Read the model definition and answer for the solid it produces. Units are mm, in the model's axes. A direction names the side the tool comes from. Give positions to 0.01 mm unless a question says otherwise; leave off trailing zeros. Write each loop counter-clockwise with the first axis right and the second up, starting at its lowest first coordinate (ties: lowest second). Pieces come first, ordered by that corner, then holes. Notation, with made-up numbers: M 5,-37 L 9,-37 A22 ccw 9,-25 Z; hole C -1.75,25.5 d2. An arc over 180 degrees is marked long. Write each question's results on one line, items separated by ' | '. Start each with the question number.
```python
from build123d import *

# Parameters (mm, degrees)
SKETCH1_R           = 2.413
SKETCH1_R_2         = 2.38125
SKETCH1_W           = 12.7
SKETCH1_H           = 3.81
BOSS_EXTRUDE1_DEPTH = 3.175
SKETCH3_W           = 292.1
SKETCH3_H           = 12.573
BOSS_EXTRUDE2_DEPTH = 8.89
BOSS_EXTRUDE3_DEPTH = 4.1275
FILLET1_R           = 2.54
FILLET2_R           = 1.27


with BuildPart() as part:
    # Sketch1 → Boss-Extrude1 (new, symmetric)
    with BuildSketch(Plane.XY):
        Polygon((-292.1, -6.2865), (-12.7, -6.2865), (-12.7, -19.05), (0, -19.05), (0, 19.05), (-12.7, 19.05), (-12.7, 6.2865), (-292.1, 6.2865), (-292.1, 8.8265), (-304.8, 19.05), (-314.96, 19.05), (-314.96, -19.05), (-304.8, -19.05), (-292.1, -8.8265), align=None)
        with Locations((-309.88, -12.7)):
            Circle(SKETCH1_R, mode=Mode.SUBTRACT)
        with Locations(Location((-309.88, 12.7, 0), (0, 0, 180))):
            Circle(SKETCH1_R, mode=Mode.SUBTRACT)
        with Locations((-6.35, 12.7)):
            Circle(SKETCH1_R_2, mode=Mode.SUBTRACT)
        with Locations(Location((-6.35, -12.7, 0), (0, 0, 180))):
            Circle(SKETCH1_R_2, mode=Mode.SUBTRACT)
        with Locations((-300.99, 3.81)):
            Rectangle(SKETCH1_W, SKETCH1_H, mode=Mode.SUBTRACT)
        with Locations((-300.99, -3.81)):
            Rectangle(SKETCH1_W, SKETCH1_H, mode=Mode.SUBTRACT)
    extrude(amount=BOSS_EXTRUDE1_DEPTH, both=True)

    # Sketch3 → Boss-Extrude2 (add)
    with BuildSketch(Plane(origin=(0, 0, -3.175), x_dir=(-1, 0, 0), z_dir=(0, 0, -1))):
        with Locations((146.05, 0)):
            Rectangle(SKETCH3_W, SKETCH3_H)
    extrude(amount=BOSS_EXTRUDE2_DEPTH)

    # Sketch4 → Boss-Extrude3 (add)
    with BuildSketch(Plane.XY.offset(3.175)):
        Polygon((-12.7, 19.05), (-63.5, 6.2865), (-12.7, 6.2865), align=None)
        Polygon((-12.7, -6.2865), (-12.7, -19.05), (-63.5, -6.2865), align=None)
    extrude(amount=-BOSS_EXTRUDE3_DEPTH)

    # Fillet1
    fillet1_edges = [part.edges().sort_by_distance(p)[0] for p in [
        (0, 19.05, 0),
        (0, -19.05, 0),
        (-292.1, -8.8265, 0),
        (-304.8, -19.05, 0),
        (-314.96, -19.05, 0),
        (-314.96, 19.05, 0),
        (-304.8, 19.05, 0),
        (-292.1, 8.8265, 0),
    ]]
    fillet(fillet1_edges, radius=FILLET1_R)

    # Fillet2
    fillet2_edges = [part.edges().sort_by_distance(p)[0] for p in [
        (0, 0, -12.065),
        (-146.05, -6.2865, -12.065),
        (-292.1, 0, -12.065),
        (-146.05, 6.2865, -12.065),
    ]]
    fillet(fillet2_edges, radius=FILLET2_R)


solid = part.part
```
Item 1: Determine the mould class of faces 5 (the cylindrical face through (-307.65, -13.62, -0.04)), 6 (the flat face through (-9, -13, -3.175)), 7 (the flat face through (-298.5, 13.98, 0.04)), 8 (the flat face through (-309, -19.05, 0)) for opening direction Y: +Y half, -Y half, draft (parallel to the pull), parting line (faces both ways), or undercut.
Item 2: Section B-B, the plane z = -7.5 is taken. Determine the outline of the cut face in (x, y).
Item 3: Section C-C, the plane x = -213.5 is taken. Determine the outline of the cut face in (y, z) (1 decimal).
Item 4: Given P1, Ø3, axis at x = -125.5, z = -10.5, coming from the +Y side; P2, Ø7, axis at x = -301.5, z = -1, coming from the -Y side; P3, Ø4, axis at x = -276, z = -6.5, coming from the -Y side; P4, Ø4.5, axis at x = -6.35, y = 12.7, coming from the +Z side, each flat-ended and moving along its own axis, determine where each tip first touches the part or whether it passes through.
Item 5: Section A-A, the plane x = -47 is taken. Determine the outline of the cut face in (y, z) (1 decimal), then the cut area to 3 significant figures.
Item 6: For faces 1 (the flat face through (-301, -5.715, 0)), 2 (the flat face through (-298.65, -14.1, 0.04)), 3 (the flat face through (-37.74, 12.76, 1.14)), 4 (the flat face through (-292.1, 0, -7)), determine the directions among +Z, -Z, +X, -X, +Y, -Y from which every point of the face is accessible in a straight line to the end or side of a thin tool.
Item 7: Straight lines are drawn through the part: line 1 (Y direction, x = -309.88, z = 0.5); line 2 (X direction, y = -3.5, z = 0); line 3 (X direction, y = -14, z = -2). For each, find the intervals that lie inside material, in ascending order.
Worked out:
1) face 5: undercut | face 6: draft | face 7: +Y half | face 8: -Y half
2) outline: M -292.1,-6.29 L 0,-6.29 L 0,6.29 L -292.1,6.29 Z
3) outline: M -6.3,-10.8 A1.3 ccw -5,-12.1 L 5,-12.1 A1.3 ccw 6.3,-10.8 L 6.3,3.2 L -6.3,3.2 Z
4) P1: stops at y = 6.29 | P2: stops at y = -18.95 | P3: stops at y = -6.29 | P4: passes through
5) outline: M -10.4,-1 L -6.3,-1 L -6.3,-10.8 A1.3 ccw -5,-12.1 L 5,-12.1 A1.3 ccw 6.3,-10.8 L 6.3,-1 L 10.4,-1 L 10.4,3.2 L -10.4,3.2 Z | area: 225 mm²
6) face 1: +Z, -Z | face 2: +Z, -Z, -Y | face 3: +Z, -Z, +Y | face 4: -Z, -X, +Y, -Y
7) line 1: y = -19.05 to -15.11, -10.29 to 10.29, 15.11 to 19.05 | line 2: x = -314.96 to -307.34, -294.64 to 0 | line 3: x = -314.96 to -311.91, -307.85 to -298.53, -12.7 to -8.35, -4.35 to 0
